from build123d import *

# Parameters (mm, degrees)
ESQUISSE1_W             = 50
ESQUISSE1_H             = 50
ESQUISSE1_R             = 2
BOSS_EXTRU_1_DEPTH      = 5
CONG_1_R                = 5
ESQUISSE2_R             = 2
ENL_V_MAT_EXTRU_1_DEPTH = 10


with BuildPart() as part:
    # Esquisse1 → Boss.-Extru.1 (new body)
    with BuildSketch(Plane(origin=(0, 0, 0), x_dir=(1, 0, 0), z_dir=(0, 1, 0))):
        Rectangle(ESQUISSE1_W, ESQUISSE1_H)
        with Locations(Location((-5, -20, 0), (0, 0, 270))):
            Circle(ESQUISSE1_R, mode=Mode.SUBTRACT)
        with Locations(Location((5, -20, 0), (0, 0, 270))):
            Circle(ESQUISSE1_R, mode=Mode.SUBTRACT)
        with Locations(Location((-5, 2, 0), (0, 0, 270))):
            Circle(ESQUISSE1_R, mode=Mode.SUBTRACT)
        with Locations(Location((5, 2, 0), (0, 0, 270))):
            Circle(ESQUISSE1_R, mode=Mode.SUBTRACT)
    extrude(amount=BOSS_EXTRU_1_DEPTH)

    # Congé1
    cong_1_edges = [part.edges().sort_by_distance(p)[0] for p in [
        (-25, 2.5, -25),
        (25, 2.5, -25),
        (25, 2.5, 25),
        (-25, 2.5, 25),
    ]]
    fillet(cong_1_edges, radius=CONG_1_R)

    # Esquisse2 → Enlèv. mat.-Extru.1 (cut)
    with BuildSketch(Plane(origin=(0, 5, 0), x_dir=(1, 0, 0), z_dir=(0, 1, 0))):
        with Locations(Location((-20, 20, 0), (0, 0, 270))):
            Circle(ESQUISSE2_R)
        with Locations(Location((-20, -20, 0), (0, 0, 270))):
            Circle(ESQUISSE2_R)
        with Locations(Location((20, -20, 0), (0, 0, 270))):
            Circle(ESQUISSE2_R)
        with Locations(Location((20, 20, 0), (0, 0, 270))):
            Circle(ESQUISSE2_R)
        with Locations(Location((-14, 13, 0), (0, 0, 270))):
            Circle(ESQUISSE2_R)
        with Locations(Location((14, 13, 0), (0, 0, 270))):
            Circle(ESQUISSE2_R)
    extrude(amount=-ENL_V_MAT_EXTRU_1_DEPTH, mode=Mode.SUBTRACT)


solid = part.part
Design review of the part built by this model. Coordinates are the model's own, in mm. Round coordinates to 2 decimals unless told otherwise and drop trailing zeros. Write each loop counter-clockwise with the first axis right and the second up, starting at its lowest first coordinate (ties: lowest second). Pieces come first, ordered by that corner, then holes.
Item 1: Consider section D-D on x = 14. Give the boundary of the cut face in (y, z).
Item 2: Draft analysis for pull direction X (two halves, no side actions). For faces 1 (the cylindrical face through (23, 3, -24)), 2 (the cylindrical face through (22, 3, -20)), 3 (the flat face through (-25, 2, 0)), 4 (the cylindrical face through (-6.2, 2.5, 18.4)), state which applies: released by +X, released by -X, zero draft, split by the parting line, or undercut.
Item 3: Consider section C-C on z = -2. Give the boundary of the cut face in (x, y), and give its area (3 significant figures).
Item 4: Consider section A-A on x = 5. Give the boundary of the cut face in (y, z), and give its area (3 significant figures).
Item 5: Consider section B-B on y = 4.25. Count the separate pieces of the cut face and the enclosed holes in it, and give its area (3 significant figures).
Item 6: For pin 1 Ø3 at (x, z) = (-14, -13) entering from +Y, flat-tipped, find the tip position at first contact; note if it passes through.
Item 7: Wall thickness on L1, parallel to X at y = 3.6, z = -13; L2, parallel to X at y = 3.6, z = -2; L3, parallel to X at y = 2.8, z = 20: over which ranges is each line inside the solid? List them lowest first.
Check values:
1. outline: (0, -25) - (5, -25) - (5, -15) - (0, -15) - close; (0, -11) - (5, -11) - (5, 25) - (0, 25) - close
2. face 1: released by +X
2. face 2: undercut
2. face 3: released by -X
2. face 4: undercut
3. outline: (-25, 0) - (-7, 0) - (-7, 5) - (-25, 5) - close; (-3, 0) - (3, 0) - (3, 5) - (-3, 5) - close; (7, 0) - (25, 0) - (25, 5) - (7, 5) - close
3. area: 210 mm2
4. outline: (0, -25) - (5, -25) - (5, -4) - (0, -4) - close; (0, 0) - (5, 0) - (5, 18) - (0, 18) - close; (0, 22) - (5, 22) - (5, 25) - (0, 25) - close
4. area: 210 mm2
5. separate pieces: 1
5. enclosed holes: 10
5. area: 2,350 mm2
6. pin 1: passes through
7. L1: x = -25 to -16, -12 to 12, 16 to 25
7. L2: x = -25 to -7, -3 to 3, 7 to 25
7. L3: x = -25 to -22, -18 to -7, -3 to 3, 7 to 18, 22 to 25
